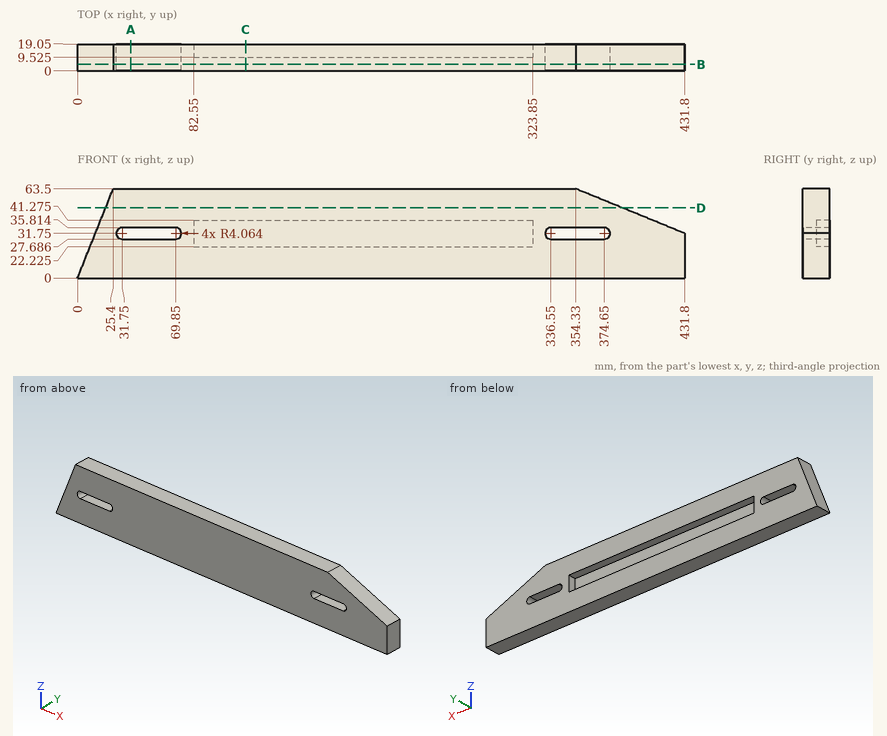
Drawing for the job (mm, zero at the part's lowest x, y, z). Give positions to 0.01 mm unless a question says otherwise; leave off trailing zeros. Order: outer loops, then holes, each group sorted by start corner. A loop starts at its lowest first (then second) coordinate and runs counter-clockwise, first axis right, second up. Notation, with made-up numbers: (72, -7.75) -> (118, -7.75) arc R30 ccw to (118, 15.25) -> close; hole circle Ø1 at (9, 48). An arc over 180 degrees is marked (long way). Use one line per item in the form item = value.
(1) Saw through at A-A (x = 38). Write the cut outline in (y, z), then the cut area to 3 significant figures.
Solution:
outline = (0, 0) -> (19.05, 0) -> (19.05, 27.69) -> (0, 27.69) -> close; (0, 35.81) -> (19.05, 35.81) -> (19.05, 63.5) -> (0, 63.5) -> close
area = 1,050 mm²
(2) Flat gauge pins, fed straight in: P1, Ø9.5, axis at x = 210, z = 33.5, coming from the +Y side (3 decimals); P2, Ø5, axis at y = 13.5, z = 35.5, coming from the -X side. Where does each tip first touch, or does it go through?
Solution:
P1 = 9.525
P2 = 13.2
(3) Saw through at B-B (y = 4.5). Write the cut outline in (x, z), then the cut area to 3 significant figures.
Solution:
outline = (0, 0) -> (431.8, 0) -> (431.8, 31.75) -> (354.33, 63.5) -> (25.4, 63.5) -> close; hole (31.75, 27.69) -> (69.85, 27.69) arc R4.06 ccw to (69.85, 35.81) -> (31.75, 35.81) arc R4.06 ccw to start; hole (336.55, 27.69) -> (374.65, 27.69) arc R4.06 ccw to (374.65, 35.81) -> (336.55, 35.81) arc R4.06 ccw to start
area = 24,700 mm²
(4) Saw through at C-C (x = 119.5). Write the cut outline in (y, z) (3 decimals).
Solution:
outline = (0, 0) -> (19.05, 0) -> (19.05, 22.225) -> (9.525, 22.225) -> (9.525, 41.275) -> (19.05, 41.275) -> (19.05, 63.5) -> (0, 63.5) -> close
(5) Saw through at D-D (z = 50). Write the cut outline in (x, y), then the cut area to 3 significant figures.
Solution:
outline = (20, 0) -> (387.27, 0) -> (387.27, 19.05) -> (20, 19.05) -> close
area = 7,000 mm²
(6) Drill centre lines: line 1 (Z direction, x = 109, y = 17.5) (3 decimals); line 2 (X direction, y = 6.5, z = 31.5); line 3 (X direction, y = 2.25, z = 28.5). Where is each one in solid material? Low to high. Write a range as from..to.
Solution:
line_1 = 0..22.225, 41.275..63.5
line_2 = 12.6..27.69, 73.91..332.49, 378.71..431.8
line_3 = 11.4..29.31, 72.29..334.11, 377.09..431.8
